The listing builds one solid part. Answer for the finished solid, in the listing's coordinates (mm). Round coordinates to 2 decimals unless told otherwise and drop trailing zeros. Loops run counter-clockwise (first coordinate to the right, second up) from the corner with the lowest first, then second, coordinate; pieces in that order, holes last. Notation, with made-up numbers: (26, -1) -> (39, -1) arc R20 ccw to (39, 16) -> close; hole circle Ø4 at (30.5, 52.5). An arc over 180 degrees is marked (long way). Write each question's results on one line, items separated by ' | '. Start each with the question number.
(1) Flat-ended cylindrical pins translate along their axes: pin 1 (3 mm diameter, centred on y = 5, z = 44, fed in from -X); pin 2 (5 mm diameter, centred on x = -11, y = 6.5, fed in from -Z); pin 3 (1 mm diameter, centred on x = -3, z = 25, fed in from +Y); pin 4 (10 mm diameter, centred on y = -8, z = 22, fed in from +X). Find the tip coordinate at first contact, or state that the pin passes through.
(2) The part is cut by section C-C (z = 18.5). Determine the outline of the cut face in (x, y), plus the area to 3 significant figures.
(3) Straight lines are drawn through the part: probe 1 along X at (y, z) = (0, 20); probe 2 along X at (y, z) = (-8.5, 30). For each, find the intervals that lie inside material, in ascending order.
(4) Determine the mould class of faces 1 (the face through (-18, 0, 0)), 2 (the face through (-3.945, -17.767, 24.65)), 3 (the face through (-3.783, -17.035, 24.65)) for opening direction Y: released by +Y, released by -Y, zero draft, split by the parting line, or undercut.
(5) The part is cut by section B-B (y = 0). Determine the outline of the cut face in (x, z).
(6) The part is cut by section A-A (x = 0). Determine the outline of the cut face in (y, z).
```python
from build123d import *

# Parameters (mm, degrees)
F0_R     = 18.2
F0_R_2   = 17.45
F1_DEPTH = 50
F3_DEPTH = 95


with BuildPart() as f1:
    # F0 (on Top) → F1 (new body)
    with BuildSketch(Plane.XY):
        Circle(F0_R)
        Circle(F0_R_2, mode=Mode.SUBTRACT)
    extrude(amount=F1_DEPTH)

    # F2 (on Front) → F3 (cut, symmetric)
    with BuildSketch(Plane.XZ):
        with BuildLine():
            ThreePointArc((10.4, 0), (0, 1.860348), (-10.4, 0))
            Line((-10.4, 0), (10.4, 0))
        make_face()
    extrude(amount=F3_DEPTH, both=True, mode=Mode.SUBTRACT)


solid = f1.part
```
Checked values:
1) pin 1: stops at x = -17.86 | pin 2: passes through | pin 3: stops at y = 18.03 | pin 4: stops at x = 17.95
2) outline: circle Ø36.4 at (0, 0); hole circle Ø34.9 at (0, 0) | area: 84.0 mm2
3) probe 1: x = -18.2 to -17.45, 17.45 to 18.2 | probe 2: x = -16.09 to -15.24, 15.24 to 16.09
4) face 1: zero draft | face 2: split by the parting line | face 3: undercut
5) outline: (-18.2, 0) -> (-17.45, 0) -> (-17.45, 50) -> (-18.2, 50) -> close; (17.45, 0) -> (18.2, 0) -> (18.2, 50) -> (17.45, 50) -> close
6) outline: (-18.2, 1.86) -> (-17.45, 1.86) -> (-17.45, 50) -> (-18.2, 50) -> close; (17.45, 1.86) -> (18.2, 1.86) -> (18.2, 50) -> (17.45, 50) -> close
